Autodesk Inventor part; units mm, degrees
ref_plane "YZ Plane" through (0, 0, 0) normal (1, 0, 0) x (0, 1, 0)
ref_plane "XZ Plane" through (0, 0, 0) normal (0, 1, 0) x (-1, 0, 0)
ref_plane "XY Plane" through (0, 0, 0) normal (0, 0, 1) x (1, 0, 0)
sketch "Sketch2" plane through (0, 0, 0) normal (0, 0, 1) x (1, 0, 0)
  line L0 (0, 0) -> (12.7, 0)
  line L1 (12.7, 0) -> (12.7, 50.8)
  line L2 (12.7, 50.8) -> (0, 50.8)
  line L3 (0, 0) -> (0, 50.8) construction
  line L4 (0, 0) -> (-12.7, 0)
  line L5 (-12.7, 0) -> (-12.7, 50.8)
  line L6 (-12.7, 50.8) -> (0, 50.8)
  dimension "d0" = 12.7
  dimension "d1" = 50.8
extrude "Extrusion1" add sketch "Sketch2" along normal mid plane 304.8
sketch "Sketch3" plane through (12.7, 0, 152.4) normal (1, 0, 0) x (0, 0, -1)
  line L0 (0, 0) -> (0, 50.8) construction
  line L1 (0, 25.4) -> (304.8, 25.4) construction
  line L2 (304.8, 50.8) -> (304.8, 0) construction
  point P0 (152.4, 0)
  point P1 (76.2, 25.4)
  point P2 (228.6, 25.4)
  point P3 (184.7909, 73.7254)
  dimension "d4" = 76.2
  dimension "d5" = 76.2
hole "Hole1" at (12.7, 25.4, 76.2) at (12.7, 25.4, -76.2) at (12.7, 73.7254, -32.3909) direction (-1, 0, 0) diameter 6.7564 end through all counterbore diameter 11.1252 counterbore depth 34.29
properties part number "RestForCuts"
Can you work these out from the model? Positions are in its coordinate system, mm. Round coordinates to 2 decimals unless told otherwise and drop trailing zeros. Loops run counter-clockwise (first coordinate to the right, second up) from the corner with the lowest first, then second, coordinate; pieces in that order, holes last. Notation, with made-up numbers: M -33.5,56.25 L -27.5,56.25 A7 cw -27.5,66.25 Z; hole C 56,60.5 d4. An arc over 180 degrees is marked long. Write item = value, one per line. Start each with the question number.
(1) If we mould it in two halves opening along Z, with no side actions, what happens to faces 1 (the face through (0, 26, -152.4)), 2 (the face through (-0.18, 20.71, -79.19)), 3 (the face through (0, 26, 152.4)), 4 (the face through (12.7, 25, -2))? For each: released by +Z, released by -Z, zero draft, split by the parting line, or undercut.
(2) I'm going to push a flat-ended pin straight in: P1, Ø10, axis at y = 25.4, z = 76.2, coming from the +X side. Where does the tip first touch, or does it pass through?
(3) I need wall thicknesses on line 1 along Z through (x, y) = (6.25, 25.4); line 2 along Y through (x, z) = (-2, 76.2). Which ranges of each line are inside material? Lowest first, please.
(4) Suppose I cut it at B-B on z = -76.2. Write out the boundary of the cut face in (x, y), plus the area to 3 significant figures.
(5) Suppose I cut it at A-A on y = 25.4. Write out the boundary of the cut face in (x, z).
Answer block:
q1.face_1 = released by -Z
q1.face_2 = undercut
q1.face_3 = released by +Z
q1.face_4 = zero draft
q2.P1 = through
q3.line_1 = -152.4 to -81.76, -70.64 to 70.64, 81.76 to 152.4
q3.line_2 = 0 to 19.84, 30.96 to 50.8
q4.outline = M -12.7,0 L 12.7,0 L 12.7,19.84 L -12.7,19.84 Z; M -12.7,30.96 L 12.7,30.96 L 12.7,50.8 L -12.7,50.8 Z
q4.area = 1,010 mm²
q5.outline = M -12.7,-152.4 L 12.7,-152.4 L 12.7,-81.76 L -12.7,-81.76 Z; M -12.7,-70.64 L 12.7,-70.64 L 12.7,70.64 L -12.7,70.64 Z; M -12.7,81.76 L 12.7,81.76 L 12.7,152.4 L -12.7,152.4 Z
